from build123d import *

# Parameters (mm, degrees)
F0_W     = 150
F0_H     = 100
F1_DEPTH = 10
F2_R     = 22.5
F3_DEPTH = 5
F4_R     = 20
F5_DEPTH = 50
F8_D     = 12
F9_D     = 12
F11_D    = 12


with BuildPart() as f1:
    # F0 (on Front) → F1 (new body)
    with BuildSketch(Plane.XZ):
        with Locations((75, -50)):
            Rectangle(F0_W, F0_H)
    extrude(amount=F1_DEPTH)

    # F2 (on face) → F3 (join)
    with BuildSketch(Plane.XZ.offset(10)):
        with Locations((75, -50)):
            Circle(F2_R)
    extrude(amount=F3_DEPTH)

    # F4 (on face) → F5 (join)
    with BuildSketch(Plane.XZ.offset(15)):
        with Locations((75, -50)):
            Circle(F4_R)
    extrude(amount=F5_DEPTH)

    # F8 (through all)
    with Locations(Plane.XZ.offset(10)):
        with Locations((136, -18)):
            Hole(F8_D / 2)

    # F9 (through all)
    with Locations(Plane.XZ.offset(10)):
        with Locations((136, -82)):
            Hole(F9_D / 2)

    # F11 (through all)
    with Locations(Plane.XZ.offset(10)):
        with Locations((14, -82), (14, -18)):
            Hole(F11_D / 2)


solid = f1.part
Could you check a few things on this model? Use its own coordinates, in mm. A direction names the side the tool comes from. Give positions to 0.01 mm unless a question says otherwise; leave off trailing zeros. Order: outer loops, then holes, each group sorted by start corner. A loop starts at its lowest first (then second) coordinate and runs counter-clockwise, first axis right, second up.
Item 1: If we section it at B-B, the plane x = 136: Write out the boundary of the cut face in (y, z), plus the area to 3 significant figures.
Item 2: If we section it at D-D, the plane x = 75: Write out the boundary of the cut face in (y, z), plus the area to 4 significant figures.
Item 3: If we section it at C-C, the plane z = -63: Write out the boundary of the cut face in (x, y), plus the area to 3 significant figures.
Item 4: If we section it at A-A, the plane z = -82: Write out the boundary of the cut face in (x, y).
Item 5: For faces 5 (the face through (94.076, -39.65, -43.993)), 6 (the face through (74, -5, -100)), which set-ups out of +Z, -Z, +X, -X, +Y, -Y let a thin tool reach every point of the face, with its end or its side?
Item 6: I need wall thicknesses on line 1 (Z direction, x = 14, y = -5); line 2 (Y direction, x = 88.5, z = -91.5); line 3 (Y direction, x = 57.5, z = -39.5). Which ranges of each line are inside material? Lowest first, please.
Item 7: I'm going to push flat-ended pins straight in: pin 1 (8 mm diameter, centred on y = -30.5, z = -43.5, fed in from +X); pin 2 (14 mm diameter, centred on x = 136, z = -18, fed in from -Y); pin 3 (1 mm diameter, centred on x = 57, y = -13, fed in from +Z); pin 4 (1 mm diameter, centred on x = 53, y = -16.5, fed in from +Z). Where does each tip first touch, or does it pass through?
Item 8: If we mould it in two halves opening along X, with no side actions, what happens to faces 1 (the face through (14.78, -4.93, -76.05)), 2 (the face through (74, 0, -49)), 3 (the face through (0, -5, -51)), 4 (the face through (57.145, -12.465, -63.691))? For each: pulls with the +X half, pulls with the -X half, needs draft (parallel to the pull), parting line crosses it, or undercut.
Values:
1. outline: (-10, -100) - (0, -100) - (0, -88) - (-10, -88) - close; (-10, -76) - (0, -76) - (0, -24) - (-10, -24) - close; (-10, -12) - (0, -12) - (0, 0) - (-10, 0) - close
1. area: 760 mm2
2. outline: (-65, -70) - (-15, -70) - (-15, -72.5) - (-10, -72.5) - (-10, -100) - (0, -100) - (0, 0) - (-10, 0) - (-10, -27.5) - (-15, -27.5) - (-15, -30) - (-65, -30) - close
2. area: 3,225 mm2
3. outline: (0, -10) - (56.64, -10) - (56.64, -15) - (59.8, -15) - (59.8, -65) - (90.2, -65) - (90.2, -15) - (93.36, -15) - (93.36, -10) - (150, -10) - (150, 0) - (0, 0) - close
3. area: 3,200 mm2
4. outline: (0, -10) - (8, -10) - (8, 0) - (0, 0) - close; (20, -10) - (130, -10) - (130, 0) - (20, 0) - close; (142, -10) - (150, -10) - (150, 0) - (142, 0) - close
5. face 5: -Y
5. face 6: -Z, +X, -X, +Y, -Y
6. line 1: z = -100 to -88, -76 to -24, -12 to 0
6. line 2: y = -10 to 0
6. line 3: y = -15 to 0
7. pin 1: stops at x = 94.84
7. pin 2: stops at y = -10
7. pin 3: stops at z = -35.86
7. pin 4: passes through
8. face 1: undercut
8. face 2: needs draft
8. face 3: pulls with the -X half
8. face 4: parting line crosses it
